```python
from build123d import *

# Parameters (mm, degrees)
SKETCH1_W               = 571.5
SKETCH1_H               = 508
BOSS_EXTRUDE1_DEPTH     = 3.175
SKETCH2_R               = 14.2875
CUT_EXTRUDE1_DEPTH      = 3.175
SKETCH4_R               = 2.0193
CUT_EXTRUDE3_DEPTH      = 1
CUT_EXTRUDE3_DEPTH_BACK = 4.175
SKETCH5_W               = 619.579537293
SKETCH5_H               = 89.035098343
CUT_EXTRUDE4_DEPTH      = 165.1


with BuildPart() as part:
    # Sketch1 → Boss-Extrude1 (new body)
    with BuildSketch(Plane(origin=(0, 0, 0), x_dir=(1, 0, 0), z_dir=(0, 1, 0))):
        with Locations((285.75, 254)):
            Rectangle(SKETCH1_W, SKETCH1_H)
    extrude(amount=BOSS_EXTRUDE1_DEPTH)

    # Sketch2 → Cut-Extrude1 (cut)
    with BuildSketch(Plane(origin=(0, 3.175, 0), x_dir=(1, 0, 0), z_dir=(0, 1, 0))):
        with Locations((330.2, 419.1)):
            Circle(SKETCH2_R)
        with Locations((330.2, 88.9)):
            Circle(SKETCH2_R)
    extrude(amount=-CUT_EXTRUDE1_DEPTH, mode=Mode.SUBTRACT)

    # Sketch4 → Cut-Extrude3 (cut, two sides)
    with BuildSketch(Plane(origin=(0, 3.175, 0), x_dir=(1, 0, 0), z_dir=(0, 1, 0))) as cut_extrude3_sk:
        with Locations((546.1, 495.3)):
            Circle(SKETCH4_R)
        with Locations((520.7, 495.3)):
            Circle(SKETCH4_R)
        with Locations((495.3, 495.3)):
            Circle(SKETCH4_R)
        with Locations((469.9, 495.3)):
            Circle(SKETCH4_R)
        with Locations((444.5, 495.3)):
            Circle(SKETCH4_R)
        with Locations((419.1, 495.3)):
            Circle(SKETCH4_R)
        with Locations((393.7, 495.3)):
            Circle(SKETCH4_R)
        with Locations((368.3, 495.3)):
            Circle(SKETCH4_R)
        with Locations((342.9, 495.3)):
            Circle(SKETCH4_R)
        with Locations((317.5, 495.3)):
            Circle(SKETCH4_R)
        with Locations((292.1, 495.3)):
            Circle(SKETCH4_R)
        with Locations((266.7, 495.3)):
            Circle(SKETCH4_R)
        with Locations((228.6, 495.3)):
            Circle(SKETCH4_R)
        with Locations((203.2, 495.3)):
            Circle(SKETCH4_R)
        with Locations((203.2, 12.7)):
            Circle(SKETCH4_R)
        with Locations((228.6, 12.7)):
            Circle(SKETCH4_R)
        with Locations((266.7, 12.7)):
            Circle(SKETCH4_R)
        with Locations((292.1, 12.7)):
            Circle(SKETCH4_R)
        with Locations((317.5, 12.7)):
            Circle(SKETCH4_R)
        with Locations((342.9, 12.7)):
            Circle(SKETCH4_R)
        with Locations((368.3, 12.7)):
            Circle(SKETCH4_R)
        with Locations((393.7, 12.7)):
            Circle(SKETCH4_R)
        with Locations((419.1, 12.7)):
            Circle(SKETCH4_R)
        with Locations((444.5, 12.7)):
            Circle(SKETCH4_R)
        with Locations((469.9, 12.7)):
            Circle(SKETCH4_R)
        with Locations((495.3, 12.7)):
            Circle(SKETCH4_R)
        with Locations((520.7, 12.7)):
            Circle(SKETCH4_R)
        with Locations((546.1, 12.7)):
            Circle(SKETCH4_R)
    extrude(amount=CUT_EXTRUDE3_DEPTH, mode=Mode.SUBTRACT)
    extrude(cut_extrude3_sk.sketch, amount=-CUT_EXTRUDE3_DEPTH_BACK, mode=Mode.SUBTRACT)

    # Sketch5 → Cut-Extrude4 (cut)
    with BuildSketch(Plane.ZY):
        with Locations((-257.641209254, 26.710529503)):
            Rectangle(SKETCH5_W, SKETCH5_H)
    extrude(amount=-CUT_EXTRUDE4_DEPTH, mode=Mode.SUBTRACT)


solid = part.part
```
Source: CAD feature listing. Evaluate the final solid. Frame: model axes, mm. Give positions to 0.01 mm unless a question says otherwise; leave off trailing zeros. Loops run counter-clockwise (first coordinate to the right, second up) from the corner with the lowest first, then second, coordinate; pieces in that order, holes last. Notation, with made-up numbers: M 32,32 L 83,32 A18 ccw 83,66 Z; hole C 70.25,29 d10. An arc over 180 degrees is marked long. Put each result on its own line as item: value.
Q1. Section B-B (z = -419.1). Return the cut outline in (x, y) (1 decimal).
Response values:
outline: M 165.1,0 L 315.9,0 L 315.9,3.2 L 165.1,3.2 Z; M 344.5,0 L 571.5,0 L 571.5,3.2 L 344.5,3.2 Z
Q2. Pin query (flat end, axial travel): P1, Ø3, axis at x = 444.5, z = -12.7, coming from the +Y side. Return the tip coordinate at first contact, or that it passes through.
Response values:
P1: passes through
Q3. Section A-A (x = 330.2). Return the cut outline in (y, z) (1 decimal).
Response values:
outline: M 0,-508 L 3.2,-508 L 3.2,-433.4 L 0,-433.4 Z; M 0,-404.8 L 3.2,-404.8 L 3.2,-103.2 L 0,-103.2 Z; M 0,-74.6 L 3.2,-74.6 L 3.2,0 L 0,0 Z
Q4. Mould query, pull axis X, two halves, no side actions, for faces 1 (the cylindrical face through (328.34, 1.61, -433.266)), 2 (the flat face through (365, 3.175, -258)). Classes: released by +X, released by -X, zero draft, split by the parting line, or undercut.
Response values:
face 1: undercut
face 2: zero draft
Q5. Line query: probe 1 along Z at (x, y) = (393.7, 1); probe 2 along Z at (x, y) = (318, 0.45); probe 3 along Z at (x, y) = (342.9, 1.85). Output: solid intervals per line, ascending. Write a range as [from, to].
Response values:
probe 1: z = [-508, -497.32], [-493.28, -14.72], [-10.68, 0]
probe 2: z = [-508, -497.26], [-493.34, -426.54], [-411.66, -96.34], [-81.46, -14.66], [-10.74, 0]
probe 3: z = [-508, -497.32], [-493.28, -425.65], [-412.55, -95.45], [-82.35, -14.72], [-10.68, 0]
